Work out the finished part from the listing and answer in its coordinate system (mm). A direction names the side the tool comes from. Coordinates: 2 decimals unless noted, no trailing zeros. Order: outer loops, then holes, each group sorted by start corner. A loop starts at its lowest first (then second) coordinate and runs counter-clockwise, first axis right, second up. Notation, with made-up numbers: M 10,63.25 L 32,63.25 A17 ccw 32,73.25 Z; hole C -5,11.25 d10. An arc over 180 degrees is marked long. Use a Markdown table: item, result.
from build123d import *

# Parameters (mm, degrees)
SKETCH_1_R      = 4.25
EXTRUDE_1_DEPTH = 2.8
FILLET_1_R      = 0.5
SKETCH_2_W      = 14
SKETCH_2_H      = 2
EXTRUDE_2_DEPTH = 1
SKETCH_3_W      = 2
SKETCH_3_H      = 14
EXTRUDE_3_DEPTH = 1
CHAMFER_1_SIZE  = 0.5
CHAMFER_2_SIZE  = 0.5
CHAMFER_3_SIZE  = 0.5


with BuildPart() as part:
    # 草图1 → 凸台-拉伸1 (new body)
    with BuildSketch(Plane(origin=(0, 0, 0), x_dir=(1, 0, 0), z_dir=(0, 1, 0))):
        with Locations(Location((0, 0, 0), (0, 0, 270))):  # turned: the seam where the file's is
            Circle(SKETCH_1_R)
    extrude(amount=EXTRUDE_1_DEPTH)

    # 圆角1
    fillet_1_edges = [part.edges().sort_by_distance(p)[0] for p in [
        (0, 2.8, -4.25),
    ]]
    fillet(fillet_1_edges, radius=FILLET_1_R)

    # 草图2 → 凸台-拉伸2 (add)
    with BuildSketch(Plane.XZ):
        Rectangle(SKETCH_2_W, SKETCH_2_H)
    extrude(amount=EXTRUDE_2_DEPTH)

    # 草图3 → 凸台-拉伸3 (add)
    with BuildSketch(Plane.XZ):
        Rectangle(SKETCH_3_W, SKETCH_3_H)
    extrude(amount=EXTRUDE_3_DEPTH)

    # 倒角1
    chamfer_1_edges = [part.edges().sort_by_distance(p)[0] for p in [
        (0, 0, 7),
    ]]
    chamfer(chamfer_1_edges, length=CHAMFER_1_SIZE)

    # 倒角2
    chamfer_2_edges = [part.edges().sort_by_distance(p)[0] for p in [
        (7, 0, 0),
    ]]
    chamfer(chamfer_2_edges, length=CHAMFER_2_SIZE)

    # 倒角3
    chamfer_3_edges = [part.edges().sort_by_distance(p)[0] for p in [
        (-7, 0, 0),
        (0, 0, -7),
    ]]
    chamfer(chamfer_3_edges, length=CHAMFER_3_SIZE)


solid = part.part
(1) A cutting plane is placed at A-A (z = 0). Determine the outline of the cut face in (x, y).
Conclusion:
| item | result |
|---|---|
| outline | M -7,-1 L 7,-1 L 7,-0.5 L 6.5,0 L 4.25,0 L 4.25,2.3 A0.5 ccw 3.75,2.8 L -3.75,2.8 A0.5 ccw -4.25,2.3 L -4.25,0 L -6.5,0 L -7,-0.5 Z |
(2) Given P1, Ø1.5, axis at x = 1.5, z = -4, coming from the +Y side; P2, Ø0.5, axis at x = -5, y = -0.5, coming from the +Z side; P3, Ø1.1, axis at y = -0.5, z = -5.5, coming from the -X side; P4, Ø2, axis at y = 2, z = -4, coming from the -X side, each flat-ended and moving along its own axis, determine where each tip first touches the part or whether it passes through.
Conclusion:
| item | result |
|---|---|
| P1 | y = 2.8 |
| P2 | z = 1 |
| P3 | x = -1 |
| P4 | x = -3.01 |
(3) A cutting plane is placed at B-B (x = 0). Determine the outline of the cut face in (y, z), then the cut area to 3 significant figures.
Conclusion:
| item | result |
|---|---|
| outline | M -1,-7 L -0.5,-7 L 0,-6.5 L 0,-4.25 L 2.3,-4.25 A0.5 ccw 2.8,-3.75 L 2.8,3.75 A0.5 ccw 2.3,4.25 L 0,4.25 L 0,6.5 L -0.5,7 L -1,7 Z |
| area | 37.4 mm2 |
(4) Which of the six approach directions +Z, -Z, +X, -X, +Y, -Y give full straight-line access (tool end or side, diameter ignored) to faces 1 (the flat face through (1, -0.5, 4)), 2 (the flat face through (-4, -0.5, -1)), 3 (the flat face through (-2, 0, 2))?
Conclusion:
| item | result |
|---|---|
| face 1 | +Z, +X, -Y |
| face 2 | -Z, -X, -Y |
| face 3 | +Z, -X, -Y |
(5) A cutting plane is placed at D-D (z = -4.5). Determine the outline of the cut face in (x, y), then the cut area to 3 significant figures.
Conclusion:
| item | result |
|---|---|
| outline | M -1,-1 L 1,-1 L 1,0 L -1,0 Z |
| area | 2.00 mm2 |
(6) Straight lines are drawn through the part: L1, parallel to Z at x = 1.5, y = -0.65; L2, parallel to Y at x = -1.5, z = 2.25; L3, parallel to Z at x = 3, y = 0.9. For each, find the intervals that lie inside material, in ascending order.
Conclusion:
| item | result |
|---|---|
| L1 | -1 to 1 |
| L2 | 0 to 2.8 |
| L3 | -3.01 to 3.01 |
(7) A cutting plane is placed at C-C (y = 0.75). Determine the outline of the cut face in (x, z).
Conclusion:
| item | result |
|---|---|
| outline | C 0,0 d8.5 |
